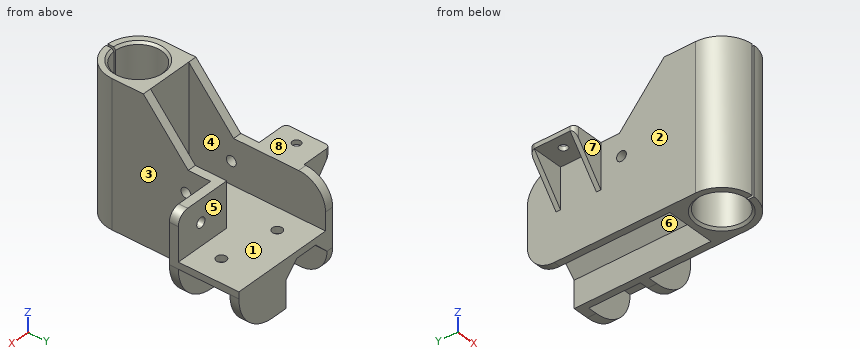
```python
from build123d import *

# Parameters (mm, degrees)
BOSS_EXTRUDE1_DEPTH     = 64
CUT_EXTRUDE1_DEPTH      = 61
CUT_EXTRUDE2_DEPTH      = 103.493902258
CUT_EXTRUDE2_DEPTH_BACK = 103.493902258
CUT_EXTRUDE3_DEPTH      = 43
CUT_EXTRUDE4_DEPTH      = 105.961897849
CHAMFER1_SIZE           = 1
SKETCH6_R               = 2.2
CUT_EXTRUDE5_DEPTH      = 94.648278148
BOSS_EXTRUDE2_DEPTH     = 14
CUT_EXTRUDE6_DEPTH      = 106.81625079
SKETCH9_R               = 1.85
CUT_EXTRUDE7_DEPTH      = 93.746967605
FILLET1_R               = 2
FILLET2_R               = 12
SKETCH10_R              = 2.2
CUT_EXTRUDE8_DEPTH      = 108.168092266
FILLET3_R               = 5
FILLET4_START           = 44
FILLET4_DEPTH           = 31
SKETCH11_R              = 2.2
CUT_EXTRUDE9_DEPTH      = 97.098348533
SKETCH12_W              = 18
SKETCH12_H              = 23
CUT_EXTRUDE10_DEPTH     = 22


with BuildPart() as part:
    # Sketch1 → Boss-Extrude1 (new body)
    with BuildSketch(Plane.XY):
        with BuildLine():
            Line((-14, 0), (-14, 75))
            Line((-14, 75), (36, 75))
            Line((36, 75), (36, 44))
            Line((36, 44), (14, 44))
            Line((14, 44), (14, 0))
            ThreePointArc((14, 0), (0, -14), (-14, 0))
        make_face()
    extrude(amount=BOSS_EXTRUDE1_DEPTH)

    # Sketch2 → Cut-Extrude1 (cut)
    with BuildSketch(Plane(origin=(0, 75, 0), x_dir=(1, 0, 0), z_dir=(0, 1, 0))):
        Polygon((-11, 0), (-11, -12), (-5, -18), (5, -18), (11, -12), (11, 0), align=None)
    extrude(amount=-CUT_EXTRUDE1_DEPTH, mode=Mode.SUBTRACT)

    # Sketch3 → Cut-Extrude2 (cut, two sides: drawn at the far end of the back side and taken through both)
    with BuildSketch(Plane(origin=(14, 0, 0), x_dir=(0, 0, -1), z_dir=(1, 0, 0)).offset(-CUT_EXTRUDE2_DEPTH_BACK)):
        Polygon((-64, 14), (-41, 34), (-41, 75), (-64, 75), align=None)
    extrude(amount=CUT_EXTRUDE2_DEPTH + CUT_EXTRUDE2_DEPTH_BACK, mode=Mode.SUBTRACT)

    # Sketch4 → Cut-Extrude3 (cut)
    with BuildSketch(Plane.XY.offset(64)):
        Polygon((-10.2, 14), (-10.2, 75), (36, 75), (36, 48), (10.2, 48), (10.2, 14), align=None)
    extrude(amount=-CUT_EXTRUDE3_DEPTH, mode=Mode.SUBTRACT)

    # Sketch5 → Cut-Extrude4 (cut, through all)
    with BuildSketch(Plane.XY.offset(64)):
        with BuildLine():
            Line((-0.5, -10.438031424), (-0.5, -13.99106858))
            ThreePointArc((-0.5, -13.99106858), (0, -14), (0.5, -13.99106858))
            Line((0.5, -13.99106858), (0.5, -10.438031424))
            ThreePointArc((0.5, -10.438031424), (0, 10.45), (-0.5, -10.438031424))
        make_face()
    extrude(amount=-CUT_EXTRUDE4_DEPTH, mode=Mode.SUBTRACT)

    # Chamfer1
    chamfer1_edges = [part.edges().sort_by_distance(p)[0] for p in [
        (0, 10.45, 0),
        (0, 10.45, 64),
    ]]
    chamfer(chamfer1_edges, length=CHAMFER1_SIZE)

    # Sketch6 → Cut-Extrude5 (cut, through all)
    with BuildSketch(Plane.XY.offset(21)):
        with Locations((0, 62)):
            Circle(SKETCH6_R)
        with Locations((0, 27)):
            Circle(SKETCH6_R)
        with Locations((25, 58)):
            Circle(SKETCH6_R)
    extrude(amount=-CUT_EXTRUDE5_DEPTH, mode=Mode.SUBTRACT)

    # Sketch7 → Boss-Extrude2 (add)
    with BuildSketch(Plane(origin=(-14, 0, 0), x_dir=(0, 0, -1), z_dir=(1, 0, 0))):
        Polygon((-41, 62.2), (-21, 62.2), (-21, 60.2), (-39, 60.2), (-39, 44.2), (-21, 44.2), (-21, 42.2), (-41, 42.2), align=None)
    extrude(amount=-BOSS_EXTRUDE2_DEPTH)

    # Sketch8 → Cut-Extrude6 (cut, through all)
    with BuildSketch(Plane(origin=(0, 62.2, 0), x_dir=(1, 0, 0), z_dir=(0, 1, 0))):
        Polygon((-14, -21), (-28, -39), (-28, -21), align=None)
    extrude(amount=-CUT_EXTRUDE6_DEPTH, mode=Mode.SUBTRACT)

    # Sketch9 → Cut-Extrude7 (cut, through all)
    with BuildSketch(Plane.XY.offset(41)):
        with Locations((-22, 52.2)):
            Circle(SKETCH9_R)
    extrude(amount=-CUT_EXTRUDE7_DEPTH, mode=Mode.SUBTRACT)

    # Fillet1
    fillet1_edges = [part.edges().sort_by_distance(p)[0] for p in [
        (-28, 42.2, 40),
        (-28, 62.2, 40),
    ]]
    fillet(fillet1_edges, radius=FILLET1_R)

    # Fillet2
    fillet2_edges = [part.edges().sort_by_distance(p)[0] for p in [
        (-12.1, 75, 41),
        (-12.5, 75, 0),
    ]]
    fillet(fillet2_edges, radius=FILLET2_R)

    # Sketch10 → Cut-Extrude8 (cut, through all)
    with BuildSketch(Plane(origin=(14, 0, 0), x_dir=(0, 0, -1), z_dir=(1, 0, 0))):
        with Locations(Location((-31, 33, 0), (0, 0, 90))):
            Circle(SKETCH10_R)
    extrude(amount=-CUT_EXTRUDE8_DEPTH, mode=Mode.SUBTRACT)

    # Fillet3
    fillet3_edges = [part.edges().sort_by_distance(p)[0] for p in [
        (36, 46, 41),
    ]]
    fillet(fillet3_edges, radius=FILLET3_R)

    # Fillet4: read off the stored shape, not the designer's step
    # Fillet4 outline → Fillet4 (cut)
    with BuildSketch(Plane(origin=(0, 0, 0), x_dir=(1, 0, 0), z_dir=(0, 1, 0)).offset(FILLET4_START)):
        with BuildLine():
            ThreePointArc((18, 0), (30.727922061, -5.272077939), (36, -18))
            Line((36, -18), (36, 0))
            Line((36, 0), (18, 0))
        make_face()
    extrude(amount=FILLET4_DEPTH, mode=Mode.SUBTRACT)

    # Sketch11 → Cut-Extrude9 (cut, through all)
    with BuildSketch(Plane(origin=(0, 48, 0), x_dir=(1, 0, 0), z_dir=(0, 1, 0))):
        with Locations(Location((24, -31, 0), (0, 0, 270))):
            Circle(SKETCH11_R)
    extrude(amount=-CUT_EXTRUDE9_DEPTH, mode=Mode.SUBTRACT)

    # Sketch12 → Cut-Extrude10 (cut)
    with BuildSketch(Plane.ZY.offset(-36)):
        with Locations((9, 59.5)):
            Rectangle(SKETCH12_W, SKETCH12_H)
    extrude(amount=CUT_EXTRUDE10_DEPTH, mode=Mode.SUBTRACT)


solid = part.part
```
CAD build for the part. Positions are in the model's coordinates, mm. Face numbers are marked on the shaded views. A direction names the side the tool comes from. Coordinates: 2 decimals unless noted, no trailing zeros. Loops run counter-clockwise (first coordinate to the right, second up) from the corner with the lowest first, then second, coordinate; pieces in that order, holes last. Notation, with made-up numbers: (-3.5, -34.5) - (30.5, -34.5) arc R22 cw to (30.5, -28.5) - close; hole circle Ø1 at (87.5, 60). An arc over 180 degrees is marked (long way). Return JSON: item names as keys, results as strings.
1. Band-saw the part on D-D (y = 52.2). Give the cut face in (x, z), and give its area (3 significant figures).
Result:
{"outline": "(-28, 39) - (-23.85, 39) - (-23.85, 41) - (-28, 41) - close; (-20.15, 39) - (-14, 39) - (-14, 0) - (-11, 0) - (-11, 12) - (-5, 18) - (5, 18) - (11, 12) - (11, 0) - (14, 0) - (14, 18) - (36, 18) - (36, 21) - (-10.2, 21) - (-10.2, 41) - (-20.15, 41) - close", "area": "391 mm2"}
2. 3-axis set-ups, long thin cutter, end or side, ignore diameter. For the marked faces 4, 5, 6, 7 and 8: which of +Z, -Z, +X, -X, +Y, -Y reach the whole face in a straight line?
Result:
{"face 4": "+Z, +Y", "face 5": "+Z, +X, +Y", "face 6": "-Z, +Y", "face 7": "+Z, -Z, -X, -Y", "face 8": "+Z, +X, -X, +Y"}
3. Band-saw the part on C-C (x = -22). Give the cut face in (y, z).
Result:
{"outline": "(42.2, 31.29) - (44.2, 31.29) - (44.2, 39) - (50.35, 39) - (50.35, 41) - (42.2, 41) - close; (54.05, 39) - (60.2, 39) - (60.2, 31.29) - (62.2, 31.29) - (62.2, 41) - (54.05, 41) - close"}
4. Mould opens along X. For the marked faces 1, 2 and 3 say: released by +X, released by -X, zero draft, split by the parting line, or undercut.
Result:
{"face 1": "undercut", "face 2": "released by -X", "face 3": "released by +X"}
5. Band-saw the part on A-A (y = 27). Give the cut face in (x, z).
Result:
{"outline": "(-14, 0) - (-11, 0) - (-11, 12) - (-5, 18) - (-2.2, 18) - (-2.2, 21) - (-10.2, 21) - (-10.2, 49.05) - (-14, 49.05) - close; (2.2, 18) - (5, 18) - (11, 12) - (11, 0) - (14, 0) - (14, 49.05) - (10.2, 49.05) - (10.2, 21) - (2.2, 21) - close"}
6. Band-saw the part on B-B (z = 25.5). Give the cut face in (x, y), and give its area (3 significant figures).
Result:
{"outline": "(-17.5, 42.2) - (-14, 42.2) - (-14, 0) arc R14 ccw to (-0.5, -13.99) - (-0.5, -10.44) arc R10.45 cw (long way) to (0.5, -10.44) - (0.5, -13.99) arc R14 ccw to (14, 0) - (14, 44) - (36, 44) - (36, 48) - (10.2, 48) - (10.2, 14) - (-10.2, 14) - (-10.2, 75) - (-14, 75) - (-14, 62.2) - (-17.5, 62.2) - (-17.5, 60.2) - (-14, 60.2) - (-14, 44.2) - (-17.5, 44.2) - close", "area": "816 mm2"}
7. Drop flat-ended pins along their axis: pin 1 (2.5 mm diameter, centred on y = 33, z = 31, fed in from -X); pin 2 (5 mm diameter, centred on x = 23.5, y = 56, fed in from -Z); pin 3 (8 mm diameter, centred on x = 5.5, z = 18.5, fed in from -Y); pin 4 (14.5 mm diameter, centred on x = -1, z = 10.5, fed in from +Y). Give the stop position or say it passes through.
Result:
{"pin 1": "passes through", "pin 2": "stops at z = 18", "pin 3": "stops at y = -13.92", "pin 4": "stops at y = 14"}
8. Probe L1, parallel to X at y = 46.15, z = 31; L2, parallel to Y at x = -22, z = 40; L3, parallel to X at y = 57, z = 3.5. List the from-to ranges inside material, lowest first. Write a range as from..to.
Result:
{"L1": "x = -14..-10.2, 10.2..21.8, 26.2..36", "L2": "y = 42.2..50.35, 54.05..62.2", "L3": "x = -14..-11, 11..14"}
